```python
from build123d import *

# Parameters (mm, degrees)
F0_R      = 20
F1_DEPTH  = 40.2
F2_R      = 20
F2_R_2    = 16.25
F3_DEPTH  = 17.8
F5_DEPTH  = 40.201
F7_R      = 13
F8_DEPTH  = 3
F10_DEPTH = 5
F11_R     = 16.25
F11_R_2   = 14
F12_DEPTH = 2.4
F14_DEPTH = 15
F18_R     = 10
F19_DEPTH = 18.4


with BuildPart() as f1:
    # F0 (on Front) → F1 (new body)
    with BuildSketch(Plane.XZ):
        Circle(F0_R)
    extrude(amount=F1_DEPTH)

    # F2 (on face) → F3 (cut)
    with BuildSketch(Plane.XZ.offset(40.2)):
        Circle(F2_R)
        Circle(F2_R_2, mode=Mode.SUBTRACT)
    extrude(amount=-F3_DEPTH, mode=Mode.SUBTRACT)

    # F4 (on face) → F5 (cut, through all)
    with BuildSketch(Plane.XZ.offset(40.2)):
        with BuildLine():
            Line((-10, 17.3205080757), (-4.7, 8.1406387956))
            ThreePointArc((-4.7, 8.1406387956), (0, -9.4), (4.7, 8.1406387956))
            Line((4.7, 8.1406387956), (10, 17.3205080757))
            ThreePointArc((10, 17.3205080757), (0, 20), (-10, 17.3205080757))
        make_face()
    extrude(amount=-F5_DEPTH, mode=Mode.SUBTRACT)

    # F7 (on offset) → F8 (cut)
    with BuildSketch(Plane.XZ.offset(33.9)):
        Circle(F7_R)
    extrude(amount=F8_DEPTH, mode=Mode.SUBTRACT)

    # F9 (on face) → F10 (cut)
    with BuildSketch(Plane.XZ.offset(40.2)):
        Polygon((11, -6.3508529611), (11, 6.3508529611), (0, 12.7017059222), (-11, 6.3508529611), (-11, -6.3508529611), (0, -12.7017059222), align=None)
    extrude(amount=-F10_DEPTH, mode=Mode.SUBTRACT)

    # F11 (on face) → F12 (cut)
    with BuildSketch(Plane.XZ.offset(40.2)):
        Circle(F11_R)
        Circle(F11_R_2, mode=Mode.SUBTRACT)
    extrude(amount=-F12_DEPTH, mode=Mode.SUBTRACT)

    # F13 (on face) → F14 (cut)
    with BuildSketch(Plane(origin=(0, 0, 0), x_dir=(-1, 0, 0), z_dir=(0, 1, 0))):
        with BuildLine():
            Line((19.9761634199, 0.9761634199), (19, 0))
            Line((19, 0), (19.9761634199, -0.9761634199))
            ThreePointArc((19.9761634199, -0.9761634199), (20, 0), (19.9761634199, 0.9761634199))
        make_face()
    extrude(amount=-F14_DEPTH, mode=Mode.SUBTRACT)

    # F15 (on Right) → F16 (revolve, cut)
    with BuildSketch(Plane.YZ):
        Polygon((-0.639097304, -20), (0, -20), (0, -19.6310169995), align=None)
    revolve(axis=Axis((0, -40.2, 0), (0, -1, 0)), mode=Mode.SUBTRACT)

    # F18 (on face) → F19 (cut)
    with BuildSketch(Plane.XZ.offset(40.2)):
        Circle(F18_R)
    extrude(amount=-F19_DEPTH, mode=Mode.SUBTRACT)

    # F20 (on Top) → F21 (revolve, cut)
    with BuildSketch(Plane.XY):
        Polygon((-10, -21.8), (-9.4, -21.8), (-9.4, -21.4535898385), align=None)
    revolve(axis=Axis((0, -40.2, 0), (0, -1, 0)), mode=Mode.SUBTRACT)


solid = f1.part
```
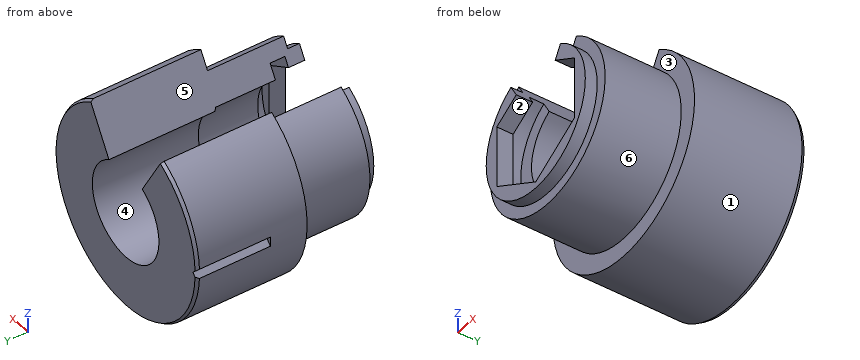
The listing builds one solid part. Answer for the finished solid, in the listing's coordinates (mm). Face numbers are marked on the shaded views. A direction names the side the tool comes from. Coordinates: 2 decimals unless noted, no trailing zeros. Write each loop counter-clockwise with the first axis right and the second up, starting at its lowest first coordinate (ties: lowest second). Pieces come first, ordered by that corner, then holes. Notation, with made-up numbers: (-37.5, 30.25) - (-8.5, 30.25) arc R34 cw to (-8.5, 60.25) - close; hole circle Ø7 at (81.5, -11.75). An arc over 180 degrees is marked (long way). Return JSON: item names as keys, results as strings. Group by question number.
Q1. Flat-ended cylindrical pins translate along their axes: pin 1 Ø1 at (y, z) = (-38, -1) entering from -X; pin 2 Ø3 at (x, z) = (15.5, -10.5) entering from -Y; pin 3 Ø7.5 at (x, z) = (2, 4.5) entering from +Y; pin 4 Ø4 at (x, y) = (-7, -5.5) entering from -Z. Find the tip coordinate at first contact, or state that the pin passes through.
Q2. For a pull along Z with two mould halves and no side action, classify the marked faces 1, 2 and 3 as +Z half, -Z half, draft (parallel to the pull), parting line (faces both ways), or undercut.
Q3. Find the intervals of material crossed by line 1 along Z through (x, y) = (0, -36.2); line 2 along Z through (x, y) = (0, -32); line 3 along Y through (x, z) = (-5, -14), in increasing order. Write a range as [from, to].
Q4. The part is cut by section A-A on y = -25.5. Write down the section's boundary in (x, z) (3 decimals).
Q5. The part is cut by section B-B on y = -18.5. Write down the section's boundary in (x, z).
Q6. Which of the six approach directions +Z, -Z, +X, -X, +Y, -Y give full straight-line access (tool end or side, diameter ignored) to the marked faces 4, 5 and 6?
Evaluation:
{
 "1": {"pin 1": "stops at x = -16.24", "pin 2": "stops at y = -22.4", "pin 3": "passes through", "pin 4": "stops at z = -19.36"},
 "2": {"face 1": "parting line", "face 2": "undercut", "face 3": "draft"},
 "3": {"line 1": "z = [-16.25, -13]", "line 2": "z = [-16.25, -10]", "line 3": "y = [-37.8, 0]"},
 "4": {"outline": "(-8.125, 14.073) arc R16.25 ccw (long way) to (8.125, 14.073) - (5, 8.66) arc R10 cw (long way) to (-5, 8.66) - close"},
 "5": {"outline": "(-10, 17.32) arc R20 ccw (long way) to (10, 17.32) - (4.7, 8.14) arc R9.4 cw (long way) to (-4.7, 8.14) - close"},
 "6": {"face 4": "+Y, -Y", "face 5": "+Z, +Y, -Y", "face 6": "-Y"}
}
